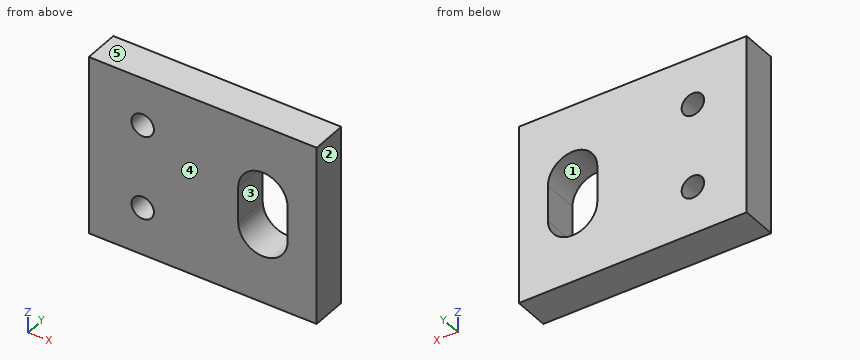
```python
from build123d import *

# Parameters (mm, degrees)
SKETCH1_W           = 25.4
SKETCH1_H           = 20
SKETCH1_R           = 1.25
BOSS_EXTRUDE1_DEPTH = 4


with BuildPart() as part:
    # Sketch1 → Boss-Extrude1 (new body)
    with BuildSketch(Plane(origin=(0, 4, 0), x_dir=(1, 0, 0), z_dir=(0, 1, 0))):
        with Locations((12.7, -10)):
            Rectangle(SKETCH1_W, SKETCH1_H)
        with Locations((6, -14.686)):
            Circle(SKETCH1_R, mode=Mode.SUBTRACT)
        with Locations((6, -5.314)):
            Circle(SKETCH1_R, mode=Mode.SUBTRACT)
        with BuildLine():
            Line((16.65, -12), (16.65, -8))
            ThreePointArc((16.65, -8), (19.4, -5.25), (22.15, -8))
            Line((22.15, -8), (22.15, -12))
            ThreePointArc((22.15, -12), (19.4, -14.75), (16.65, -12))
        make_face(mode=Mode.SUBTRACT)
    extrude(amount=-BOSS_EXTRUDE1_DEPTH)


solid = part.part
```
Source: CAD feature listing. Evaluate the final solid. Frame: model axes, mm. Face numbers are marked on the shaded views. A direction names the side the tool comes from. Coordinates: 2 decimals unless noted, no trailing zeros. Loops run counter-clockwise (first coordinate to the right, second up) from the corner with the lowest first, then second, coordinate; pieces in that order, holes last. Notation, with made-up numbers: M 88.5,87 L 128.5,87 A20 ccw 128.5,110 Z; hole C -27,-31 d2. An arc over 180 degrees is marked long. Use a Markdown table: item, result. Add a question column.
Q1. Material intervals for L1, parallel to Z at x = 6, y = 1.45; L2, parallel to X at y = 1.25, z = 14.25; L3, parallel to X at y = 1.8, z = 9, sorted ascending.
Q2. Section query D-D, the plane y = 3. Return loops of the section in (x, z), and give its area (3 significant figures).
Q3. Section query C-C, the plane x = 19.4. Return loops of the section in (y, z).
Q4. Draft query along Z for the marked faces 3, 4 and 5. Return one class per face: pulls with the +Z half, pulls with the -Z half, needs draft (parallel to the pull), parting line crosses it, or undercut.
Q5. Section query B-B, the plane z = 15.5. Return loops of the section in (x, y), and give its area (3 significant figures).
Q6. Section query A-A, the plane x = 6. Return loops of the section in (y, z), and give its area (3 significant figures).
Q7. Access query for the marked faces 1 and 2. Directions: +Z, -Z, +X, -X, +Y, -Y. A direction counts if a zero-diameter tool reaches every point of the face in a straight line with its end or side. Return the directions, or none.
Result:
| question | item | result |
|---|---|---|
| 1 | L1 | z = 0 to 4.06, 6.56 to 13.44, 15.94 to 20 |
| 1 | L2 | x = 0 to 4.83, 7.17 to 17.82, 20.98 to 25.4 |
| 1 | L3 | x = 0 to 16.65, 22.15 to 25.4 |
| 2 | outline | M 0,0 L 25.4,0 L 25.4,20 L 0,20 Z; hole C 6,5.31 d2.5; hole C 6,14.69 d2.5; hole M 16.65,8 A2.75 ccw 22.15,8 L 22.15,12 A2.75 ccw 16.65,12 Z |
| 2 | area | 452 mm2 |
| 3 | outline | M 0,0 L 4,0 L 4,5.25 L 0,5.25 Z; M 0,14.75 L 4,14.75 L 4,20 L 0,20 Z |
| 4 | face 3 | undercut |
| 4 | face 4 | needs draft |
| 4 | face 5 | pulls with the +Z half |
| 5 | outline | M 0,0 L 5.05,0 L 5.05,4 L 0,4 Z; M 6.95,0 L 25.4,0 L 25.4,4 L 6.95,4 Z |
| 5 | area | 94.0 mm2 |
| 6 | outline | M 0,0 L 4,0 L 4,4.06 L 0,4.06 Z; M 0,6.56 L 4,6.56 L 4,13.44 L 0,13.44 Z; M 0,15.94 L 4,15.94 L 4,20 L 0,20 Z |
| 6 | area | 60.0 mm2 |
| 7 | face 1 | +Y, -Y |
| 7 | face 2 | +Z, -Z, +X, +Y, -Y |
